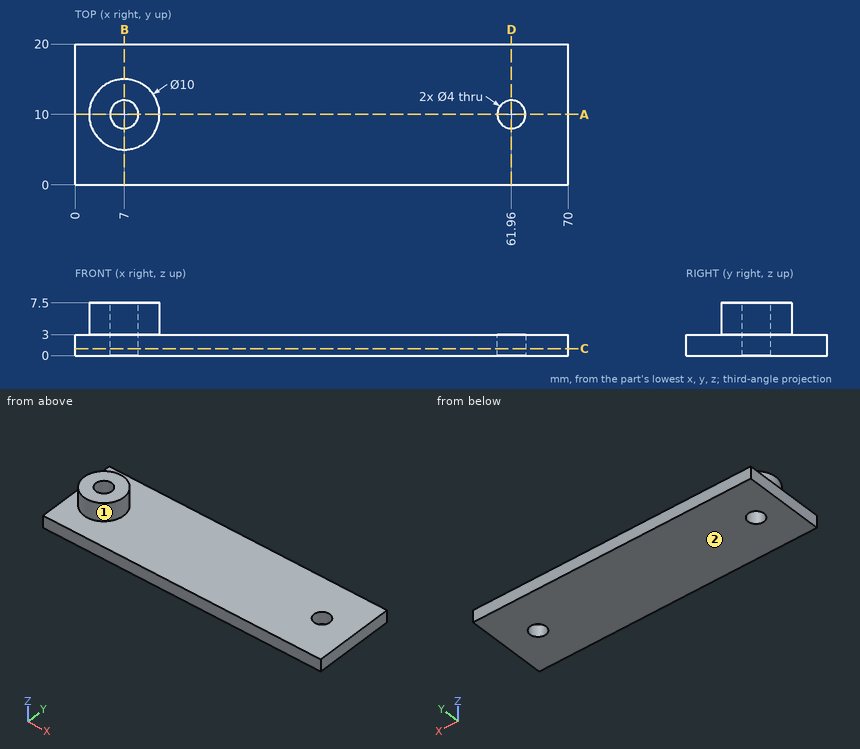
Study the drawing (mm; zero at the part's minimum x, y, z) and answer. A direction names the side the tool comes from. Round coordinates to 2 decimals unless told otherwise and drop trailing zeros. Write each loop counter-clockwise with the first axis right and the second up, starting at its lowest first coordinate (ties: lowest second). Pieces come first, ordered by that corner, then holes. Notation, with made-up numbers: (58.5, 33) - (110.5, 33) arc R28 ccw to (110.5, 70) - close; hole circle Ø7 at (-33.75, 46.25). An arc over 180 degrees is marked (long way). Use a Markdown table: item, result. Add a question column.
1. The part is cut by section C-C (z = 1). Write down the section's boundary in (x, y).
2. The part is cut by section B-B (x = 7). Write down the section's boundary in (y, z), and give its area (3 significant figures).
3. A tool of negligible diameter and unlimited length cuts with its end or side. For the marked faces 1 and 2, from which of +Z, -Z, +X, -X, +Y, -Y can it reach the whole face along a straight path? Write none if from no direction.
4. The part is cut by section A-A (y = 10). Write down the section's boundary in (x, z), and give its area (3 significant figures).
5. Flat-ended cylindrical pins translate along their axes: P1, Ø12, axis at x = 32.5, y = 11.5, coming from the +Z side; P2, Ø3, axis at x = 7, y = 10, coming from the +Z side. Find the tip coordinate at first contact, or state that the pin passes through.
6. Consider line 1 (Y direction, x = 61.96, z = 1.95); line 2 (Z direction, x = 47.5, y = 4); line 3 (X direction, y = 9.75, z = 6.25). Determine where each line is inside the solid, lowest interval first.
7. The part is cut by section D-D (x = 61.96). Write down the section's boundary in (y, z), and give its area (3 significant figures).
Reported:
| question | item | result |
|---|---|---|
| 1 | outline | (0, 0) - (70, 0) - (70, 20) - (0, 20) - close; hole circle Ø4 at (7, 10); hole circle Ø4 at (61.96, 10) |
| 2 | outline | (0, 0) - (8, 0) - (8, 7.5) - (5, 7.5) - (5, 3) - (0, 3) - close; (12, 0) - (20, 0) - (20, 3) - (15, 3) - (15, 7.5) - (12, 7.5) - close |
| 2 | area | 75.0 mm^2 |
| 3 | face 1 | +Z |
| 3 | face 2 | -Z, +X, -X, +Y, -Y |
| 4 | outline | (0, 0) - (5, 0) - (5, 7.5) - (2, 7.5) - (2, 3) - (0, 3) - close; (9, 0) - (59.96, 0) - (59.96, 3) - (12, 3) - (12, 7.5) - (9, 7.5) - close; (63.96, 0) - (70, 0) - (70, 3) - (63.96, 3) - close |
| 4 | area | 213 mm^2 |
| 5 | P1 | z = 3 |
| 5 | P2 | through |
| 6 | line 1 | 0 to 8, 12 to 20 |
| 6 | line 2 | 0 to 3 |
| 6 | line 3 | 2.01 to 5.02, 8.98 to 11.99 |
| 7 | outline | (0, 0) - (8, 0) - (8, 3) - (0, 3) - close; (12, 0) - (20, 0) - (20, 3) - (12, 3) - close |
| 7 | area | 48.0 mm^2 |
